Autodesk Inventor part; units mm, degrees
ref_plane "YZ Plane" through (0, 0, 0) normal (1, 0, 0) x (0, 1, 0)
ref_plane "XZ Plane" through (0, 0, 0) normal (0, 1, 0) x (-1, 0, 0)
ref_plane "XY Plane" through (0, 0, 0) normal (0, 0, 1) x (1, 0, 0)
sketch "Sketch1" plane through (0, 0, 0) normal (0, 1, 0) x (-1, 0, 0)
  line L0 (0, 0) -> (60, 0)
  line L1 (60, 0) -> (60, -30)
  line L2 (60, -30) -> (30, -30)
  line L3 (30, -30) -> (30, -60)
  line L4 (30, -60) -> (0, -60)
  line L5 (0, -60) -> (0, 0)
  dimension "d0" = 60
  dimension "d1" = 30
  dimension "d2" = 30
  dimension "d3" = 30
  dimension "d4" = 30
extrude "Extrusion1" add sketch "Sketch1" along normal blind 15
sketch "Sketch13" plane through (0, 0, 0) normal (0, -1, 0) x (1, 0, 0)
  circle A0 centre (-4, -4) radius 1.5
  circle A1 centre (-26, -4) radius 1.5
  circle A2 centre (-4, -26) radius 1.5
  circle A3 centre (-26, -26) radius 1.5
  point P0 (0, 0)
  dimension "d55" = 3
  dimension "d56" = 3
  dimension "d57" = 3
  dimension "d58" = 3
extrude "Extrusion7" cut sketch "Sketch13" against normal up to next
sketch "Sketch14" plane through (0, 0, 0) normal (0, -1, 0) x (1, 0, 0)
  circle A0 centre (-41, -15) radius 1.5
  line L0 (-60, 0) -> (-60, -30)
  line L1 (0, 0) -> (-60, 0)
  circle A1 centre (-15, -45) radius 3
  line L2 (-30, -60) -> (0, -60)
  line L3 (-30, -30) -> (-30, -60)
  dimension "d61" = 3
  dimension "d62" = 19
  dimension "d63" = 15
  dimension "d64" = 6
  dimension "d65" = 15
  dimension "d66" = 15
extrude "Extrusion8" cut sketch "Sketch14" against normal up to next
sketch "Sketch15" plane through (0, 0, 0) normal (0, -1, 0) x (1, 0, 0)
  circle A0 centre (-15, -45) radius 5.5
  point P0 (0, 0)
  dimension "d69" = 11
extrude "Extrusion9" cut sketch "Sketch15" against normal blind 11
sketch "Sketch2" plane through (0, 0, 0) normal (0, -1, 0) x (1, 0, 0)
  point P0 (-15, -45)
sketch "Sketch3" plane through (0, 15, 0) normal (0, 1, 0) x (1, 0, 0)
  point P0 (-45, 15)
properties part number "wooden1" material "Aluminum 6061"
Source: CAD feature listing. Evaluate the final solid. Frame: model axes, mm. A direction names the side the tool comes from. Round coordinates to 2 decimals unless told otherwise and drop trailing zeros. Order: outer loops, then holes, each group sorted by start corner. A loop starts at its lowest first (then second) coordinate and runs counter-clockwise, first axis right, second up. Notation, with made-up numbers: (65.25, -30) -> (105.25, -30) arc R24 cw to (105.25, -13) -> close; hole circle Ø1 at (-1, 82). An arc over 180 degrees is marked (long way). One line per item, written item: value. Start each with the question number.
Q1. Access query for faces 1 (the cylindrical face through (-2.57, 7.4, -3.55)), 2 (the flat face through (-30, 7, -45)), 3 (the flat face through (-12.6, 11, -47.4)). Directions: +Z, -Z, +X, -X, +Y, -Y. A direction counts if a zero-diameter tool reaches every point of the face in a straight line with its end or side. Return the directions, or none.
Q2. Pin query (flat end, axial travel): pin 1 (9 mm diameter, centred on x = -15, z = -45, fed in from -Y); pin 2 (5.5 mm diameter, centred on x = -15, z = -45, fed in from -Y). Return the tip coordinate at first contact, or that it passes through.
Q3. Section query C-C (x = -4). Return the cut outline in (y, z).
Q4. Material intervals for probe 1 along Z at (x, y) = (-4, 5); probe 2 along Z at (x, y) = (-15, 12); probe 3 along Z at (x, y) = (-38.5, 3), sorted ascending.
Q5. Section query B-B (z = -15). Return the cut outline in (x, y), plus the area to 3 significant figures.
Q6. Section query D-D (y = 1.25). Return the cut outline in (x, z).
Q7. Section query A-A (x = -15). Return the cut outline in (y, z).
Q8. Draft query along X for faces 4 (the flat face through (-15, 7, -60)), 5 (the flat face through (-60, 7, -15)), 6 (the cylindrical face through (-27.5, 7.4, -3.93)). Return one class per face: pulls with the +X half, pulls with the -X half, needs draft (parallel to the pull), parting line crosses it, or undercut.
Findings below:
1. face 1: +Y, -Y
1. face 2: -Z, -X, +Y, -Y
1. face 3: -Y
2. pin 1: y = 11
2. pin 2: through
3. outline: (0, -60) -> (15, -60) -> (15, -27.5) -> (0, -27.5) -> close; (0, -24.5) -> (15, -24.5) -> (15, -5.5) -> (0, -5.5) -> close; (0, -2.5) -> (15, -2.5) -> (15, 0) -> (0, 0) -> close
4. probe 1: -60 to -27.5, -24.5 to -5.5, -2.5 to 0
4. probe 2: -60 to -48, -42 to 0
4. probe 3: -30 to 0
5. outline: (-60, 0) -> (-42.5, 0) -> (-42.5, 15) -> (-60, 15) -> close; (-39.5, 0) -> (0, 0) -> (0, 15) -> (-39.5, 15) -> close
5. area: 855 mm²
6. outline: (-60, -30) -> (-30, -30) -> (-30, -60) -> (0, -60) -> (0, 0) -> (-60, 0) -> close; hole circle Ø3 at (-41, -15); hole circle Ø3 at (-26, -26); hole circle Ø3 at (-26, -4); hole circle Ø11 at (-15, -45); hole circle Ø3 at (-4, -26); hole circle Ø3 at (-4, -4)
7. outline: (0, -60) -> (15, -60) -> (15, -48) -> (11, -48) -> (11, -50.5) -> (0, -50.5) -> close; (0, -39.5) -> (11, -39.5) -> (11, -42) -> (15, -42) -> (15, 0) -> (0, 0) -> close
8. face 4: needs draft
8. face 5: pulls with the -X half
8. face 6: undercut
